Check sheet for the modelled part. Datum: model origin and axes. Units: mm. Face numbers are marked on the shaded views. Round coordinates to 2 decimals unless told otherwise and drop trailing zeros. Order: outer loops, then holes, each group sorted by start corner. A loop starts at its lowest first (then second) coordinate and runs counter-clockwise, first axis right, second up.
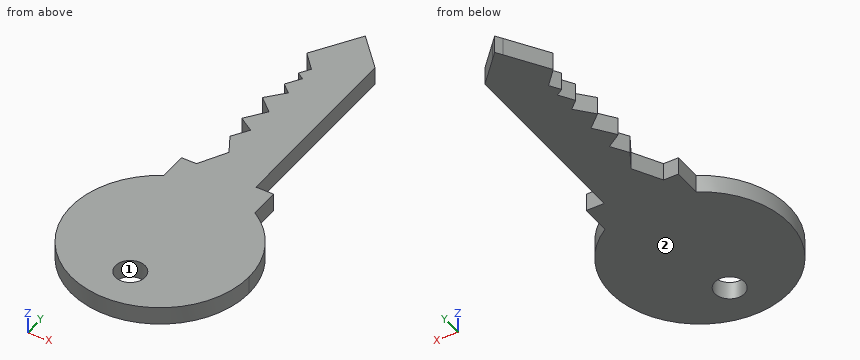
from build123d import *

# Parameters (mm, degrees)
F0_R     = 2
F1_DEPTH = 2.4


with BuildPart() as f1:
    # F0 (on Top) → F1 (new body)
    with BuildSketch(Plane.XY):
        Polygon((-5.955262, 15.422773), (-8, 11.712709), (-4.8, 11.712709), (-4.554067, 40.688071), (-8, 35.361156), (-6, 33.171624), (-6.895736, 31.786946), (-5.955262, 31.178562), (-7.199531, 29.255102), (-5.955262, 28.143108), (-8, 25.855143), (-6, 24.067757), (-8, 21.422476), (-6, 20.128694), (-7.410005, 17.94903), align=None)
        Polygon((-3.2, 11.712709), (0, 11.712709), (0, 37.262041), (-3.2, 40.688071), align=None)
        with BuildLine():
            Line((-10, 11.712709), (-10, 7.936883))
            ThreePointArc((-10, 7.936883), (-7.105829, 9.135688), (-4, 9.544578))
            Line((-4, 9.544578), (-4, 11.712709))
            Line((-4, 11.712709), (-4.8, 11.712709))
            Line((-4.8, 11.712709), (-8, 11.712709))
            Line((-8, 11.712709), (-10, 11.712709))
        make_face()
        with BuildLine():
            ThreePointArc((-4, 9.544578), (-0.66911, 9.073029), (2.4, 7.69544))
            Line((2.4, 7.69544), (2.4, 11.712709))
            Line((2.4, 11.712709), (0, 11.712709))
            Line((0, 11.712709), (-3.2, 11.712709))
            Line((-3.2, 11.712709), (-4, 11.712709))
            Line((-4, 11.712709), (-4, 9.544578))
        make_face()
        with BuildLine():
            ThreePointArc((-10, 7.936883), (-10, -12.847727), (8, -2.455422))
            ThreePointArc((8, -2.455422), (6.50714, 3.341129), (2.4, 7.69544))
            ThreePointArc((2.4, 7.69544), (-0.66911, 9.073029), (-4, 9.544578))
            ThreePointArc((-4, 9.544578), (-7.105829, 9.135688), (-10, 7.936883))
        make_face()
        with Locations((-4, -8.855422)):
            Circle(F0_R, mode=Mode.SUBTRACT)
        Polygon((-4, 41.544578), (-4, 11.712709), (-3.2, 11.712709), (-3.2, 40.688071), align=None)
        Polygon((-4.8, 11.712709), (-4, 11.712709), (-4, 41.544578), (-4.554067, 40.688071), align=None)
    extrude(amount=F1_DEPTH)


solid = f1.part
1) Gauge pin test, flat end, axial feed: pin 1 (0.7 mm diameter, centred on y = 10, z = 1, fed in from +X). Record the tip position at first contact, or that the pin passes through.
2) Scan lines: line 1 (X direction, y = -9.5, z = 1.5); line 2 (Y direction, x = -7, z = 1); line 3 (X direction, y = 11, z = 1.4). Record each from-to range of solid material in increasing order.
3) Draft check along Y on the marked faces 1 and 2. Enter one of: pulls with the +Y half, pulls with the -Y half, needs draft (parallel to the pull), parting line crosses it, or undercut.
4) Sectioned sample at B-B on y = 8.5. Record the cut outline in (x, z), and give its area (3 significant figures).
5) Sectioned sample at C-C on y = 38. Record the cut outline in (x, z).
6) Sectioned sample at A-A on z = 1.6. Record the cut outline in (x, y), and give its area (3 significant figures).
Values found:
1. pin 1: stops at x = 2.4
2. line 1: x = -13.71 to -5.89, -2.11 to 5.71
2. line 2: y = -14.07 to 13.53, 17.24 to 18.58, 20.78 to 22.75, 24.96 to 26.97, 29.08 to 29.56, 34.27 to 36.91
2. line 3: x = -10 to 2.4
3. face 1: undercut
3. face 2: needs draft
4. outline: (-10, 0) - (2.4, 0) - (2.4, 2.4) - (-10, 2.4) - close
4. area: 29.8 mm2
5. outline: (-6.29, 0) - (-0.69, 0) - (-0.69, 2.4) - (-6.29, 2.4) - close
6. outline: (-10, 7.94) arc R12 ccw (long way) to (8, -2.46) arc R12 ccw to (2.4, 7.7) - (2.4, 11.71) - (0, 11.71) - (0, 37.26) - (-3.2, 40.69) - (-4, 41.54) - (-4.55, 40.69) - (-8, 35.36) - (-6, 33.17) - (-6.9, 31.79) - (-5.96, 31.18) - (-7.2, 29.26) - (-5.96, 28.14) - (-8, 25.86) - (-6, 24.07) - (-8, 21.42) - (-6, 20.13) - (-7.41, 17.95) - (-5.96, 15.42) - (-8, 11.71) - (-10, 11.71) - close; hole circle Ø4 at (-4, -8.86)
6. area: 664 mm2
